The model under review builds one solid part; all positions refer to its coordinate system, in mm. A direction names the side the tool comes from. Give positions to 0.01 mm unless a question says otherwise; leave off trailing zeros. Loops run counter-clockwise (first coordinate to the right, second up) from the corner with the lowest first, then second, coordinate; pieces in that order, holes last. Notation, with made-up numbers: M 67,85 L 72,85 A17 cw 72,90 Z; hole C 21.5,63 d2. An arc over 180 degrees is marked long. Write item = value, one per line. Start each with the question number.
1. For faces 1 (the face through (-14, -3, 0)), 2 (the face through (-27, -3.175, -150)), list the 3-axis set-ups (+Z, -Z, +X, -X, +Y, -Y) from which the entire face can be reached by the end or side of a thin tool; tool diameter is ignored.
2. Wall thickness on line 1 along X through (y, z) = (-1.85, -38.1); line 2 along Z through (x, y) = (-1, -25); line 3 along X through (y, z) = (-43.5, -64.5) (3 decimals): over which ranges is each line inside the solid? List them lowest first. Write a range as from..to.
3. For pin 1 (10 mm diameter, centred on x = -24, z = -49.5, fed in from +Y); pin 2 (10.5 mm diameter, centred on y = -25.4, z = -38.1, fed in from -X) (3 decimals); pin 3 (1 mm diameter, centred on x = -26, z = -182.5, fed in from -Y) (3 decimals); pin 4 (7 mm diameter, centred on x = -25.4, z = -38.1, fed in from -Y), all flat-tipped, find the tip position at first contact; note any pin that passes through.
4. We need section D-D on z = -171.5. Give the boundary of the cut face in (x, y) (3 decimals), then the cut area to 3 significant figures.
5. Draft analysis for pull direction X (two halves, no side actions). For faces 3 (the face through (-1.57, -21.62, -36.91)), 4 (the face through (-21.62, -1.57, -36.91)), 5 (the face through (-3.175, -27, -150)), state which applies: pulls with the +X half, pulls with the -X half, needs draft (parallel to the pull), parting line crosses it, or undercut.
6. We need section A-A on x = -25.4. Give the boundary of the cut face in (y, z) (3 decimals).
7. We need section B-B on z = -38.1. Give the boundary of the cut face in (x, y) (3 decimals).
from build123d import *

# Parameters (mm, degrees)
F1_DEPTH = 304.8
F2_R     = 3.9624
F3_DEPTH = 50.801
F4_R     = 3.9624
F5_DEPTH = 50.801


with BuildPart() as f1:
    # F0 (on Top) → F1 (new body)
    with BuildSketch(Plane.XY):
        Polygon((0, 0), (-50.8, 0), (-50.8, -3.175), (-3.175, -3.175), (-3.175, -50.795514), (0, -50.8), align=None)
    extrude(amount=-F1_DEPTH)

    # F2 (on Right) → F3 (cut, through all)
    with BuildSketch(Plane.YZ):
        with Locations((-25.4, -38.1)):
            Circle(F2_R)
    extrude(amount=-F3_DEPTH, mode=Mode.SUBTRACT)

    # F4 (on Front) → F5 (cut, through all)
    with BuildSketch(Plane.XZ):
        with Locations((-25.4, -38.1)):
            Circle(F4_R)
    extrude(amount=F5_DEPTH, mode=Mode.SUBTRACT)


solid = f1.part
Final values:
q1.face_1 = +Z, +X, -X, +Y, -Y
q1.face_2 = +Z, -Z, -X, -Y
q2.line_1 = -50.8..-29.36, -21.44..0
q2.line_2 = -304.8..-42.04, -34.16..0
q2.line_3 = -3.175..0
q3.pin_1 = 0
q3.pin_2 = -3.175
q3.pin_3 = -3.175
q3.pin_4 = through
q4.outline = M -50.8,-3.175 L -3.175,-3.175 L -3.175,-50.796 L 0,-50.8 L 0,0 L -50.8,0 Z
q4.area = 312 mm²
q5.face_3 = needs draft
q5.face_4 = undercut
q5.face_5 = pulls with the -X half
q6.outline = M -3.175,-304.8 L 0,-304.8 L 0,-42.062 L -3.175,-42.062 Z; M -3.175,-34.138 L 0,-34.138 L 0,0 L -3.175,0 Z
q7.outline = M -50.8,-3.175 L -29.362,-3.175 L -29.362,0 L -50.8,0 Z; M -21.438,-3.175 L -3.175,-3.175 L -3.175,-21.438 L 0,-21.438 L 0,0 L -21.438,0 Z; M -3.175,-50.796 L 0,-50.8 L 0,-29.362 L -3.175,-29.362 Z
